Geometry check sheet. Reference: the model listing, model coordinates, mm. A direction names the side the tool comes from. Round coordinates to 2 decimals unless told otherwise and drop trailing zeros. Write each loop counter-clockwise with the first axis right and the second up, starting at its lowest first coordinate (ties: lowest second). Pieces come first, ordered by that corner, then holes.
from build123d import *

# Parameters (mm, degrees)
EXTRUDE_1_DEPTH      = 2
EXTRUDE_1_DEPTH_BACK = 1
SKETCH_1_W           = 31.2
SKETCH_1_H           = 24
EXTRUDE_2_DEPTH      = 36
EXTRUDE_2_DEPTH_BACK = 3
SKETCH_2_W           = 31.2
SKETCH_2_H           = 4
SKETCH_3_R           = 1.4
EXTRUDE_3_DEPTH      = 3
SKETCH_4_R           = 1.4
CUT_EXTRUDE_1_DEPTH  = 8
SKETCH_5_W           = 17
SKETCH_5_H           = 1
CUT_EXTRUDE_2_DEPTH  = 31.2
CUT_EXTRUDE_3_DEPTH  = 31.2
SKETCH_7_R           = 1.4
EXTRUDE_4_DEPTH      = 4


with BuildPart() as part:
    # 草图1 → 凸台-拉伸1 (new, two sides: drawn at the far end of the back side and taken through both)
    with BuildSketch(Plane.XY.offset(-EXTRUDE_1_DEPTH_BACK)):
        Rectangle(SKETCH_1_W, SKETCH_1_H)
    extrude(amount=EXTRUDE_1_DEPTH + EXTRUDE_1_DEPTH_BACK)

    # 草图2 → 凸台-拉伸2 (add, two sides: drawn at the far end of the back side and taken through both)
    with BuildSketch(Plane.XY.offset(2).offset(-EXTRUDE_2_DEPTH_BACK)):
        with Locations((0, 14)):
            Rectangle(SKETCH_2_W, SKETCH_2_H)
        with Locations((0, -14)):
            Rectangle(SKETCH_2_W, SKETCH_2_H)
    extrude(amount=EXTRUDE_2_DEPTH + EXTRUDE_2_DEPTH_BACK)

    # 草图3 → 凸台-拉伸3 (add)
    # profile 1 of 2: a face of its own
    with BuildSketch(Plane.ZY.offset(15.6)):
        Polygon((38, 16), (31, 16), (22.152932489, 16), (32.310715372, 6), (38, 6), align=None)
        with Locations((34, 9)):
            Circle(SKETCH_3_R, mode=Mode.SUBTRACT)
    # profile 2 of 2: a face of its own
    with BuildSketch(Plane.ZY.offset(15.6)):
        Polygon((38, -16), (38, -6), (32.310715372, -6), (22.152932489, -16), (31, -16), align=None)
        with Locations(Location((34, -9, 0), (0, 0, 180))):
            Circle(SKETCH_3_R, mode=Mode.SUBTRACT)
    extrude_3 = extrude(amount=EXTRUDE_3_DEPTH)

    # 草图4 → 切除-拉伸1 (cut)
    with BuildSketch(Plane(origin=(0, 0, -1), x_dir=(-1, 0, 0), z_dir=(0, 0, -1))):
        with Locations((13.6, -14)):
            Circle(SKETCH_4_R)
        with Locations(Location((13.6, 14, 0), (0, 0, 180))):
            Circle(SKETCH_4_R)
        with Locations(Location((-13.6, -14, 0), (0, 0, 180))):
            Circle(SKETCH_4_R)
        with Locations((-13.6, 14)):
            Circle(SKETCH_4_R)
    extrude(amount=-CUT_EXTRUDE_1_DEPTH, mode=Mode.SUBTRACT)

    # 镜向1: 凸台-拉伸3 across plane
    add(extrude_3.mirror(Plane(origin=(0, 0, 0), x_dir=(0, 0, 1), z_dir=(1, 0, 0))))

    # 草图5 → 切除-拉伸2 (cut)
    with BuildSketch(Plane.ZY.offset(15.6)):
        with Locations((27.5, 12.5)):
            Rectangle(SKETCH_5_W, SKETCH_5_H)
        with Locations((27.5, -12.5)):
            Rectangle(SKETCH_5_W, SKETCH_5_H)
    extrude(amount=-CUT_EXTRUDE_2_DEPTH, mode=Mode.SUBTRACT)

    # 草图6 → 切除-拉伸3 (cut)
    with BuildSketch(Plane.ZY.offset(15.6)):
        Polygon((1.3, 0), (1.5, 12), (2, 12), (2, -12), (1.5, -12), align=None)
    extrude(amount=-CUT_EXTRUDE_3_DEPTH, mode=Mode.SUBTRACT)

    # 草图7 → 凸台-拉伸4 (add)
    # profile 1 of 2: a face of its own
    with BuildSketch(Plane.XY.offset(38)):
        Polygon((-15.6, 12), (15.6, 12), (15.6, 16), (15.6, 21), (-15.6, 21), (-15.6, 16), align=None)
        with Locations((-10, 18.5)):
            Circle(SKETCH_7_R, mode=Mode.SUBTRACT)
        with Locations(Location((10, 18.5, 0), (0, 0, 180))):
            Circle(SKETCH_7_R, mode=Mode.SUBTRACT)
    # profile 2 of 2: a face of its own
    with BuildSketch(Plane.XY.offset(38)):
        Polygon((-15.6, -16), (-15.6, -21), (15.6, -21), (15.6, -16), (15.6, -12), (-15.6, -12), align=None)
        with Locations((10, -18.5)):
            Circle(SKETCH_7_R, mode=Mode.SUBTRACT)
        with Locations(Location((-10, -18.5, 0), (0, 0, 180))):
            Circle(SKETCH_7_R, mode=Mode.SUBTRACT)
    extrude(amount=EXTRUDE_4_DEPTH)


solid = part.part
1. Access from +Z, -Z, +X, -X, +Y, -Y to the whole of each face (thin tool, end or side, straight path). Record for faces 4 (the face through (0, 19, 38)), 5 (the face through (0, -16, 18)), 6 (the face through (15.6, -17, 40)), 7 (the face through (14.35, -15.18, 2.94)), 8 (the face through (15.6, -10.2, 32.9)).
2. Scan lines: line 1 along Y through (x, z) = (-12, 19.5); line 2 along Z through (x, y) = (-8, -12.5); line 3 along Y through (x, z) = (6.5, 2). Record each from-to range of solid material in increasing order.
3. Section check B-B (z = 13). Record the cut outline in (x, y), plus the area to 3 significant figures.
4. Depth check by flat-ended pin: pin 1 Ø2.5 at (x, y) = (13.6, 14) entering from -Z; pin 2 Ø3 at (x, y) = (13.5, -13.5) entering from -Z; pin 3 Ø5 at (x, z) = (6.5, 4.5) entering from +Y; pin 4 Ø5 at (x, y) = (-4, -8) entering from +Z (3 decimals). Enter the tip coordinate at first touch or a pass-through.
5. Release check for a two-part mould opening along Z. For faces 1 (the face through (-17.08, 9.06, 32.6)), 2 (the face through (-17.08, 11.07, 27.16)), 3 (the face through (17, 6, 35)) record: +Z half, -Z half, draft (parallel to the pull), parting line (faces both ways), or undercut.
6. Section check A-A (x = 10). State how many separate pieces and enclosed holes the cut face has, plus the area to 3 significant figures.
7. Section check C-C (y = 18.5). Record the cut outline in (x, z).
Results below:
1. face 4: -Z, +X, -X, +Y
1. face 5: -Z, +X, -X, -Y
1. face 6: +Z, +X, +Y, -Y
1. face 7: -Z
1. face 8: none
2. line 1: y = -16 to -13, 13 to 16
2. line 2: z = -1 to 19, 36 to 42
2. line 3: y = -16 to -12, 12 to 16
3. outline: (-15.6, -16) - (15.6, -16) - (15.6, -12) - (-15.6, -12) - close; (-15.6, 12) - (15.6, 12) - (15.6, 16) - (-15.6, 16) - close
3. area: 250 mm2
4. pin 1: stops at z = 7
4. pin 2: stops at z = -1
4. pin 3: stops at y = 16
4. pin 4: stops at z = 1.475
5. face 1: undercut
5. face 2: -Z half
5. face 3: draft
6. separate pieces: 3
6. enclosed holes: 0
6. area: 385 mm2
7. outline: (-15.6, 38) - (-11.4, 38) - (-11.4, 42) - (-15.6, 42) - close; (-8.6, 38) - (8.6, 38) - (8.6, 42) - (-8.6, 42) - close; (11.4, 38) - (15.6, 38) - (15.6, 42) - (11.4, 42) - close
